The listing builds one solid part. Answer for the finished solid, in the listing's coordinates (mm). A direction names the side the tool comes from. Coordinates: 2 decimals unless noted, no trailing zeros. Order: outer loops, then holes, each group sorted by start corner. A loop starts at its lowest first (then second) coordinate and runs counter-clockwise, first axis right, second up. Notation, with made-up numbers: (18.25, 62) - (77.25, 62) arc R24 ccw to (77.25, 84) - close; hole circle Ø2 at (25, -12.5). An arc over 180 degrees is marked (long way). Use a Markdown table: item, result. Add a question column.
Item 1: Find the intervals of material crossed by line 1 along X through (y, z) = (8, 4.35); line 2 along X through (y, z) = (1.5, 0.3); line 3 along Z through (x, y) = (44, -3.5), in increasing order.
Item 2: The mould has two halves that part along Y. Classify faces 4 (the flat face through (34.75, -9, 1)), 5 (the flat face through (49, 0, 6)), 6 (the flat face through (23, -17.5, 2)), 7 (the cylindrical face through (-17.08, 12.63, 1.48)): released by +Y, released by -Y, zero draft, split by the parting line, or undercut.
Item 3: The part is cut by section D-D, the plane x = 27. Give the vertices of the cut face in (y, z), then the cut area to 3 significant figures.
Item 4: The part is cut by section B-B, the plane z = 2.3. Give the vertices of the cut face in (x, y) (3 decimals), then the cut area to 3 significant figures.
Item 5: For faces 1 (the flat face through (12, 0, 3)), 2 (the cylindrical face through (-17.38, -12.365, 1.479)), 3 (the cylindrical face through (36.339, 4.875, 1.479)), determine the directions among +Z, -Z, +X, -X, +Y, -Y from which every point of the face is accessible in a straight line to the end or side of a thin tool.
Item 6: The part is cut by section C-C, the plane y = -11. Give the vertices of the cut face in (x, z).
Item 7: The part is cut by section A-A, the plane x = -14.32. Give the vertices of the cut face in (y, z).
Item 8: Flat-ended cylindrical pins translate along their axes: P1, Ø2.5, axis at y = -3, z = 4, coming from the -X side; P2, Ø5.5, axis at x = -14.32, y = 0, coming from the +Z side; P3, Ø3.5, axis at y = 9, z = 2, coming from the -X side. Find the tip coordinate at first contact, or state that the pin passes through.
from build123d import *

# Parameters (mm, degrees)
SKETCH_1_R      = 1.65
EXTRUDE_1_DEPTH = 3
FILLET_1_R      = 20
SKETCH_4_W      = 3
SKETCH_4_H      = 35
EXTRUDE_2_DEPTH = 6


with BuildPart() as part:
    # 草图1 → 凸台-拉伸1 (new body)
    with BuildSketch(Plane.XY):
        Polygon((0, 17.5), (50, 17.5), (50, -17.5), (0, -17.5), (-24, -17.5), (-24, 17.5), align=None)
        with Locations((36.375, 0)):
            Circle(SKETCH_1_R, mode=Mode.SUBTRACT)
        with Locations((-14.32, 0)):
            Circle(SKETCH_1_R, mode=Mode.SUBTRACT)
        with BuildLine():
            Line((34.75, 12.5), (34.75, 6.5))
            ThreePointArc((34.75, 6.5), (36.375, 4.875), (38, 6.5))
            Line((38, 6.5), (38, 12.5))
            ThreePointArc((38, 12.5), (36.375, 14.125), (34.75, 12.5))
        make_face(mode=Mode.SUBTRACT)
        with BuildLine():
            Line((34.75, -6.5), (34.75, -12.5))
            ThreePointArc((34.75, -12.5), (36.375, -14.125), (38, -12.5))
            Line((38, -12.5), (38, -6.5))
            ThreePointArc((38, -6.5), (36.375, -4.875), (34.75, -6.5))
        make_face(mode=Mode.SUBTRACT)
    extrude(amount=EXTRUDE_1_DEPTH)

    # 圆角1
    # the kernel refuses this fillet: 20 mm, written as the material it takes off along each edge
    with BuildSketch(Plane(origin=(-24, -17.5, -50), x_dir=(1, 0, 0), z_dir=(0, 0, 1))) as fillet_1_piece_1:
        with BuildLine():
            CenterArc((FILLET_1_R, FILLET_1_R), FILLET_1_R, 180, 90)
            Line((0, FILLET_1_R), (0, 0))
            Line((0, 0), (FILLET_1_R, 0))
        make_face()
    extrude(amount=103, mode=Mode.SUBTRACT)
    with BuildSketch(Plane(origin=(-24, 17.5, -50), x_dir=(1, 0, 0), z_dir=(0, 0, 1))) as fillet_1_piece_2:
        with BuildLine():
            CenterArc((FILLET_1_R, -FILLET_1_R), FILLET_1_R, 90, 90)
            Line((0, -FILLET_1_R), (0, 0))
            Line((0, 0), (FILLET_1_R, 0))
        make_face()
    extrude(amount=103, mode=Mode.SUBTRACT)

    # 草图4 → 凸台-拉伸2 (add)
    with BuildSketch(Plane(origin=(0, 0, 0), x_dir=(-1, 0, 0), z_dir=(0, 0, -1))):
        with Locations((-48.5, 0)):
            Rectangle(SKETCH_4_W, SKETCH_4_H)
    extrude(amount=-EXTRUDE_2_DEPTH)


solid = part.part
Solution:
| question | item | result |
|---|---|---|
| 1 | line 1 | x = 47 to 50 |
| 1 | line 2 | x = -23.6 to -15.01, -13.63 to 35.69, 37.06 to 50 |
| 1 | line 3 | z = 0 to 3 |
| 2 | face 4 | undercut |
| 2 | face 5 | zero draft |
| 2 | face 6 | released by -Y |
| 2 | face 7 | released by +Y |
| 3 | outline | (-17.5, 0) - (17.5, 0) - (17.5, 3) - (-17.5, 3) - close |
| 3 | area | 105 mm2 |
| 4 | outline | (-23.843, 0) arc R20 ccw to (-4, -17.5) - (50, -17.5) - (50, 17.5) - (-4, 17.5) arc R20 ccw to start; hole circle Ø3.3 at (-14.32, 0); hole circle Ø3.3 at (36.375, 0); hole (34.75, -12.5) arc R1.625 ccw to (38, -12.5) - (38, -6.5) arc R1.625 ccw to (34.75, -6.5) - close; hole (34.75, 6.5) arc R1.625 ccw to (38, 6.5) - (38, 12.5) arc R1.625 ccw to (34.75, 12.5) - close |
| 4 | area | 2,350 mm2 |
| 5 | face 1 | +Z, -X, +Y, -Y |
| 5 | face 2 | +Z, -Z, -X, -Y |
| 5 | face 3 | +Z, -Z |
| 6 | outline | (-18.76, 0) - (34.75, 0) - (34.75, 3) - (-18.76, 3) - close; (38, 0) - (50, 0) - (50, 6) - (47, 6) - (47, 3) - (38, 3) - close |
| 7 | outline | (-14.63, 0) - (-1.65, 0) - (-1.65, 3) - (-14.63, 3) - close; (1.65, 0) - (14.63, 0) - (14.63, 3) - (1.65, 3) - close |
| 8 | P1 | stops at x = -23.43 |
| 8 | P2 | stops at z = 3 |
| 8 | P3 | stops at x = -21.46 |
